```python
from build123d import *

# Parameters (mm, degrees)
F0_R     = 1.5875
F1_DEPTH = 3.175
F3_DEPTH = 101.6
F4_R     = 2.38125
F5_DEPTH = 31.751


with BuildPart() as f1:
    # F0 (on Front) → F1 (new body)
    with BuildSketch(Plane.XZ):
        with BuildLine():
            Line((-47.625, 0), (-3.175, 0))
            ThreePointArc((-3.175, 0), (-0.929936, 0.929936), (0, 3.175))
            Line((0, 3.175), (0, 152.4))
            ThreePointArc((0, 152.4), (-0.929936, 154.645064), (-3.175, 155.575))
            Line((-3.175, 155.575), (-47.625, 155.575))
            ThreePointArc((-47.625, 155.575), (-49.870064, 154.645064), (-50.8, 152.4))
            Line((-50.8, 152.4), (-50.8, 3.175))
            ThreePointArc((-50.8, 3.175), (-49.870064, 0.929936), (-47.625, 0))
        make_face()
        with Locations((-38.1, 19.05)):
            Circle(F0_R, mode=Mode.SUBTRACT)
        with Locations((-12.7, 19.05)):
            Circle(F0_R, mode=Mode.SUBTRACT)
        with Locations((-38.1, 136.525)):
            Circle(F0_R, mode=Mode.SUBTRACT)
        with Locations((-12.7, 136.525)):
            Circle(F0_R, mode=Mode.SUBTRACT)
    extrude(amount=-F1_DEPTH)

    # F2 (on face) → F3 (join)
    with BuildSketch(Plane(origin=(0, 3.175, 0), x_dir=(-1, 0, 0), z_dir=(0, 1, 0))):
        with BuildLine():
            ThreePointArc((27.517005, 24.217467), (28.298458, 23.147245), (28.575, 21.851264))
            Line((28.575, 21.851264), (28.575, 6.35))
            ThreePointArc((28.575, 6.35), (25.4, 3.175), (22.225, 6.35))
            Line((22.225, 6.35), (22.225, 21.850242))
            ThreePointArc((22.225, 21.850242), (22.501635, 23.14643), (23.283333, 24.216747))
            ThreePointArc((23.283333, 24.216747), (23.674183, 24.751906), (23.8125, 25.4))
            ThreePointArc((23.8125, 25.4), (22.873094, 26.849183), (21.166667, 26.583253))
            ThreePointArc((21.166667, 26.583253), (19.60327, 24.442619), (19.05, 21.850242))
            Line((19.05, 21.850242), (19.05, 6.35))
            ThreePointArc((19.05, 6.35), (25.4, 0), (31.75, 6.35))
            Line((31.75, 6.35), (31.75, 21.851264))
            ThreePointArc((31.75, 21.851264), (31.197009, 24.443019), (29.634349, 26.583366))
            ThreePointArc((29.634349, 26.583366), (27.927668, 26.849523), (26.988262, 25.4))
            ThreePointArc((26.988262, 25.4), (27.126467, 24.752321), (27.517005, 24.217467))
        make_face()
    extrude(amount=F3_DEPTH)

    # F4 (on face) → F5 (cut, through all)
    with BuildSketch(Plane.YZ.offset(-19.05)):
        with Locations((15.875, 14.100121)):
            Circle(F4_R)
        with Locations((92.075, 14.100121)):
            Circle(F4_R)
    extrude(amount=-F5_DEPTH, mode=Mode.SUBTRACT)


solid = f1.part
```
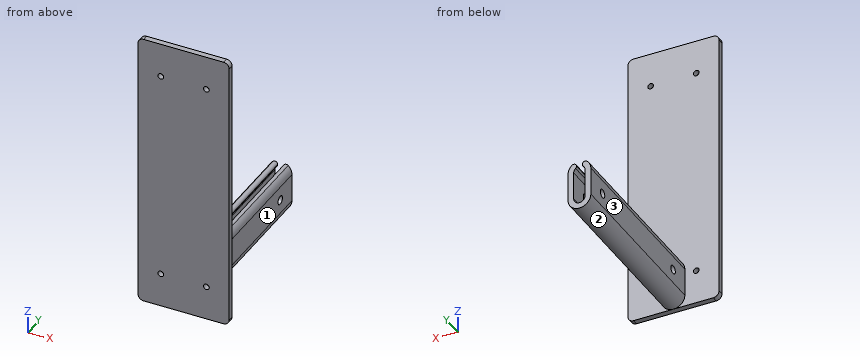
Verification items for the finished model (mm, model axes). Face numbers are marked on the shaded views. A direction names the side the tool comes from. Round coordinates to 2 decimals unless told otherwise and drop trailing zeros. Write each loop counter-clockwise with the first axis right and the second up, starting at its lowest first coordinate (ties: lowest second). Pieces come first, ordered by that corner, then holes. Notation, with made-up numbers: (9, 31) -> (21, 31) arc R23 cw to (21, 66) -> close; hole circle Ø2 at (75, 35.5). An arc over 180 degrees is marked (long way). Write each question's results on one line, items separated by ' | '. Start each with the question number.
1. Material ranges on probe 1 along X at (y, z) = (1, 19); probe 2 along X at (y, z) = (66, 10) (3 decimals); probe 3 along Y at (x, z) = (-12, 122.5) (3 decimals), recorded low to high. Write a range as from..to.
2. Set-up check for the marked faces 1, 2 and 3: record each of +Z, -Z, +X, -X, +Y, -Y from which the full face is reachable in a straight line by a thin tool's end or side.
3. Cross-section at B-B (x = -38.1). Enter the section's corners in (y, z) (1 decimal), then the cut area to 3 significant figures.
4. Cross-section at A-A (z = 19.05). Count the separate pieces of the cut face and the enclosed holes in it, then the cut area to 3 significant figures.
5. Depth check by flat-ended pin: P1, Ø7.5, axis at y = 15.88, z = 14.1, coming from the +X side; P2, Ø12.5, axis at y = 66, z = 13, coming from the -X side; P3, Ø4, axis at x = -38.1, z = 136.525, coming from the +Y side (3 decimals); P4, Ø10, axis at x = -40.5, z = 128.5, coming from the -Y side. Enter the tip coordinate at first touch or a pass-through.
Solutions:
1) probe 1: x = -50.8..-39.69, -36.51..-14.29, -11.11..0 | probe 2: x = -31.75..-28.575, -22.225..-19.05 | probe 3: y = 0..3.175
2) face 1: +Z, -Z, +X, +Y | face 2: -Z, +Y | face 3: +Z, -Z, -X, +Y
3) outline: (0, 0) -> (3.2, 0) -> (3.2, 17.5) -> (0, 17.5) -> close; (0, 20.6) -> (3.2, 20.6) -> (3.2, 134.9) -> (0, 134.9) -> close; (0, 138.1) -> (3.2, 138.1) -> (3.2, 155.6) -> (0, 155.6) -> close | area: 474 mm2
4) separate pieces: 3 | enclosed holes: 0 | area: 786 mm2
5) P1: stops at x = -19.05 | P2: stops at x = -31.75 | P3: stops at y = 3.175 | P4: stops at y = 0
